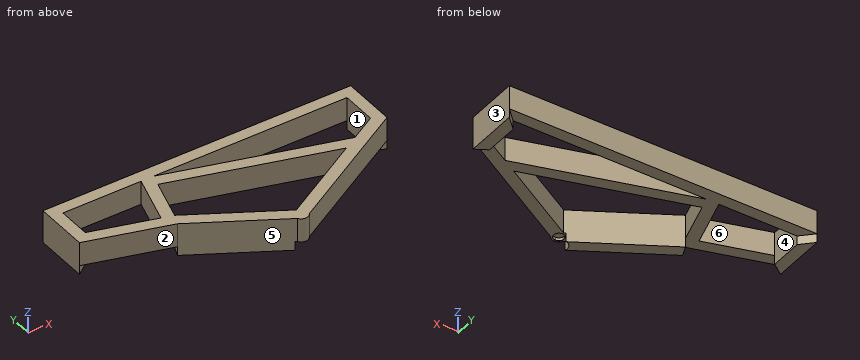
from build123d import *

# Parameters (mm, degrees)
SKETCH_6_W          = 80
SKETCH_6_H          = 40
SKETCH_6_W_2        = 76
SKETCH_6_H_2        = 36
SKETCH_14_W         = 40
SKETCH_14_H         = 80
EXTRUDE_1_DEPTH     = 194
SKETCH_15_W         = 80
SKETCH_15_H         = 40
EXTRUDE_2_DEPTH     = 595
EXTRUDE_3_DEPTH     = 30
SKETCH_17_R         = 23.094010768
EXTRUDE_4_DEPTH     = 110
SKETCH_18_R         = 27.5
SKETCH_18_R_2       = 23.094010768
CUT_EXTRUDE_1_DEPTH = 30
SKETCH_22_R         = 23.094010768
CUT_EXTRUDE_3_DEPTH = 30
CUT_EXTRUDE_4_DEPTH = 10
FILLET_1_R          = 0.5


with BuildPart() as part:
    # По траектории13: sweep along a curve in space
    with BuildLine() as sweep_13_path:
        Line((0, 0, 0), (1000, 0, 0))
        Line((1000, 0, 0), (1000, -150, 0))
        Line((1000, -150, 0), (566.987298108, -400, 0))
        Line((566.987298108, -400, 0), (263.878406783, -225, 0))
        Line((263.878406783, -225, 0), (0, -147.584326952, 0))
        Line((0, -147.584326952, 0), (0, 0, 0))
    # Эскиз6 → По траектории13 (sweep)
    with BuildSketch(Plane(origin=(0, 0, 0), x_dir=(0, 0, -1), z_dir=(1, 0, 0))):
        with Locations((-0.551773823, -1.216505436)):
            Rectangle(SKETCH_6_W, SKETCH_6_H)
        with Locations((-0.551773823, -1.216505436)):
            Rectangle(SKETCH_6_W_2, SKETCH_6_H_2, mode=Mode.SUBTRACT)
    sweep(path=sweep_13_path.line, transition=Transition.RIGHT)

    # Эскиз14 → Бобышка-Вытянуть1 (add)
    with BuildSketch(Plane(origin=(-33.89376203, -115.529989888, 0), x_dir=(0.9595578428480989, -0.2815115383580276, 0), z_dir=(0.2815115383580276, 0.9595578428480989, 0))):
        with Locations((299.085913187, -0.551773823)):
            Rectangle(SKETCH_14_W, SKETCH_14_H)
    extrude(amount=EXTRUDE_1_DEPTH)

    # Эскиз15 → Бобышка-Вытянуть2 (add)
    with BuildSketch(Plane(origin=(306.181390541, -89.82636629, 0), x_dir=(0, 0, -1), z_dir=(0.9595578428480989, -0.28151153835802767, 0))):
        with Locations((-0.551773823, 51.50143726)):
            Rectangle(SKETCH_15_W, SKETCH_15_H)
    extrude(amount=EXTRUDE_2_DEPTH)

    # Эскиз16 → Бобышка-Вытянуть3 (add)
    with BuildSketch(Plane(origin=(0, 0, -39.448226177), x_dir=(-1, 0, 0), z_dir=(0, 0, -1))):
        Polygon((18.783494564, 18.783494564), (18.783494564, -161.648850746), (-21.216505436, -131.698036755), (-21.216505436, -21.216505436), align=None)
        Polygon((-272.28762851, -205.356356178), (-256.433515773, -242.391001456), (-566.987298108, -421.689311285), (-566.987298108, -375.50128975), align=None)
        Polygon((-1018.783494564, 18.783494564), (-978.783494564, -21.216505436), (-978.783494564, -137.750644875), (-1018.783494564, -160.844655643), align=None)
    extrude(amount=EXTRUDE_3_DEPTH)

    # Эскиз17 → Бобышка-Вытянуть4 (add)
    with BuildSketch(Plane(origin=(0, 0, -69.448226177), x_dir=(-1, 0, 0), z_dir=(0, 0, -1))):
        with Locations((-566.987298108, -398.595300518)):
            Circle(SKETCH_17_R)
    extrude(amount=-EXTRUDE_4_DEPTH)

    # Эскиз18 → Вырез-Вытянуть1 (cut)
    with BuildSketch(Plane(origin=(0, 0, -69.448226177), x_dir=(-1, 0, 0), z_dir=(0, 0, -1))):
        with Locations((-566.987298108, -398.595300518)):
            Circle(SKETCH_18_R)
        with Locations((-566.987298108, -398.595300518)):
            Circle(SKETCH_18_R_2, mode=Mode.SUBTRACT)
    extrude(amount=-CUT_EXTRUDE_1_DEPTH, mode=Mode.SUBTRACT)

    # Эскиз22 → Вырез-Вытянуть3 (cut)
    with BuildSketch(Plane(origin=(0, 0, -69.448226177), x_dir=(-1, 0, 0), z_dir=(0, 0, -1))):
        with Locations((-566.987298108, -398.595300518)):
            Circle(SKETCH_22_R)
    extrude(amount=-CUT_EXTRUDE_3_DEPTH, mode=Mode.SUBTRACT)

    # Эскиз23 → Вырез-Вытянуть4 (cut)
    with BuildSketch(Plane(origin=(0, 0, -39.448226177), x_dir=(-1, 0, 0), z_dir=(0, 0, -1))):
        with BuildLine():
            ThreePointArc((-549.487298108, -398.595300518), (-554.612929437, -386.220931847), (-566.987298108, -381.095300518))
            Line((-566.987298108, -381.095300518), (-566.987298108, -416.095300518))
            ThreePointArc((-566.987298108, -416.095300518), (-554.612929437, -410.969669189), (-549.487298108, -398.595300518))
        make_face()
        with BuildLine():
            Line((-566.987298108, -416.095300518), (-566.987298108, -381.095300518))
            ThreePointArc((-566.987298108, -381.095300518), (-584.487298108, -398.595300518), (-566.987298108, -416.095300518))
        make_face()
    extrude(amount=-CUT_EXTRUDE_4_DEPTH, mode=Mode.SUBTRACT)

    # Скругление1
    fillet_1_edges = [part.edges().sort_by_distance(p)[0] for p in [
        (566.987298108, -416.095300518, -39.448226177),
    ]]
    fillet(fillet_1_edges, radius=FILLET_1_R)


solid = part.part
Can you work these out from the model? Positions are in its coordinate system, mm. Face numbers are marked on the shaded views. A direction names the side the tool comes from. Coordinates: 2 decimals unless noted, no trailing zeros. Write each loop counter-clockwise with the first axis right and the second up, starting at its lowest first coordinate (ties: lowest second). Pieces come first, ordered by that corner, then holes. Notation, with made-up numbers: (9.5, 61) -> (38.5, 61) arc R17 cw to (38.5, 72) -> close; hole circle Ø1 at (16.25, 1). An arc over 180 degrees is marked (long way). Write each question's results on one line, items separated by ' | '. Start each with the question number.
Item 1: Please list where these lines run through material, in increasing order: probe 1 along Y at (x, z) = (734, -29); probe 2 along Y at (x, z) = (184, 31); probe 3 along Y at (x, z) = (866, -20.5).
Item 2: On a 3-axis mill with a long thin cutter (end or side, diameter ignored), from which of +Z, -Z, +X, -X, +Y, -Y can I reach the whole of each face in a straight line? I mean the marked faces 5 and 6. Say none if no direction works.
Item 3: If we section it at D-D, the plane z = -55: Write out the boundary of the cut face in (x, y).
Item 4: If we section it at C-C, the plane y = -104: Write out the boundary of the cut face in (x, z).
Item 5: If we section it at B-B, the plane x = 114: Write out the boundary of the cut face in (y, z), and give its area (3 significant figures).
Item 6: Thinking about a two-plate mould opening in Y: for the marked faces 1, 2, 3 and 4, which applies, released by +Y, released by -Y, zero draft, split by the parting line, or undercut?
Item 7: I'm going to push flat-ended pins straight in: P1, Ø1.5, axis at y = -345, z = -31.5, coming from the -X side; P2, Ø10, axis at y = -288, z = 0.5, coming from the -X side; P3, Ø2, axis at y = -225.5, z = -49.5, coming from the +X side. Where does each tip first touch, or does it pass through?
Item 8: If we section it at A-A, the plane x = 406.5: Write out the boundary of the cut face in (y, z), and give its area (3 significant figures).
Answer block:
1) probe 1: -325.26 to -322.96, -281.39 to -279.08, -182.51 to -140.82, -21.22 to -19.22, 16.78 to 18.78 | probe 2: -221.14 to -219.06, -181.54 to -179.45, -21.22 to -19.22, 16.78 to 18.78 | probe 3: -249.05 to -246.74, -221.23 to -179.55, -21.22 to -19.22, 16.78 to 18.78
2) face 5: +Z, -Z, -X, -Y | face 6: +Z, -Z
3) outline: (-18.78, -161.65) -> (21.22, -131.7) -> (21.22, -21.22) -> (-18.78, 18.78) -> close; (256.43, -242.39) -> (540.64, -406.48) arc R27.5 cw to (560.64, -371.84) -> (272.29, -205.36) -> close; (978.78, -137.75) -> (1018.78, -160.84) -> (1018.78, 18.78) -> (978.78, -21.22) -> close
4) outline: (-18.78, -69.45) -> (21.22, -69.45) -> (21.22, 40.55) -> (-18.78, 40.55) -> close; (260.34, -39.45) -> (302.02, -39.45) -> (302.02, 40.55) -> (260.34, 40.55) -> close; (466.39, -39.45) -> (608.48, -39.45) -> (608.48, 40.55) -> (466.39, 40.55) -> close; (978.78, -69.45) -> (1018.78, -69.45) -> (1018.78, 40.55) -> (978.78, 40.55) -> close; hole (-16.78, -37.45) -> (19.22, -37.45) -> (19.22, 38.55) -> (-16.78, 38.55) -> close; hole (980.78, -37.45) -> (1016.78, -37.45) -> (1016.78, 38.55) -> (980.78, 38.55) -> close
5) outline: (-200.6, -39.45) -> (-158.92, -39.45) -> (-158.92, 40.55) -> (-200.6, 40.55) -> close; (-21.22, -39.45) -> (18.78, -39.45) -> (18.78, 40.55) -> (-21.22, 40.55) -> close; hole (-198.52, -37.45) -> (-161, -37.45) -> (-161, 38.55) -> (-198.52, 38.55) -> close; hole (-19.22, -37.45) -> (16.78, -37.45) -> (16.78, 38.55) -> (-19.22, 38.55) -> close | area: 948 mm²
6) face 1: undercut | face 2: released by -Y | face 3: zero draft | face 4: undercut
7) P1: x = 432.86 | P2: x = 326.77 | P3: x = 308.91
8) outline: (-329.03, -69.45) -> (-282.84, -69.45) -> (-282.84, 40.55) -> (-329.03, 40.55) -> close; (-86.43, -39.45) -> (-44.74, -39.45) -> (-44.74, 40.55) -> (-86.43, 40.55) -> close; (-21.22, -39.45) -> (18.78, -39.45) -> (18.78, 40.55) -> (-21.22, 40.55) -> close; hole (-326.72, -37.45) -> (-285.15, -37.45) -> (-285.15, 38.55) -> (-326.72, 38.55) -> close; hole (-19.22, -37.45) -> (16.78, -37.45) -> (16.78, 38.55) -> (-19.22, 38.55) -> close | area: 5,720 mm²
